Geometry check sheet. Reference: the model listing, model coordinates, mm. Coordinates: 2 decimals unless noted, no trailing zeros. Write each loop counter-clockwise with the first axis right and the second up, starting at its lowest first coordinate (ties: lowest second). Pieces come first, ordered by that corner, then holes. Notation, with made-up numbers: (33.5, -6.5) -> (53.5, -6.5) arc R23 cw to (53.5, 31.5) -> close; hole circle Ø11 at (87.25, -0.75). An arc over 180 degrees is marked (long way). One line per question, with ' | ' between items.
from build123d import *

# Parameters (mm, degrees)
KREISMUSTER1_COUNT = 15


with BuildPart() as part:
    # Skizze1 → Rotation1 (revolve)
    with BuildSketch(Plane.XY, mode=Mode.PRIVATE) as rotation1_sk:
        Polygon((16.14475863, 0), (16.14475863, 8.608081897), (23.261403386, 8.608081897), (28.845024076, 5.234644397), (28.845024076, 0), align=None)
    revolve(rotation1_sk.sketch.rotate(Axis((0, 0, 0), (0, 1, 0)), 90), axis=Axis((0, 0, 0), (0, 1, 0)))  # turned: the seam where the file's is

    # Skizze2 → Schnitt-Rotation1 (revolve, cut)
    with BuildSketch(Plane.XY):
        Polygon((18.433980943, 12.441833146), (35.219041201, 3.611138793), (33.767638602, 0.852365915), (16.982578344, 9.683060267), align=None)
    schnitt_rotation1 = revolve(axis=Axis((14.262929412, 14.636241782, 0), (0.884995308, -0.465599941, 0)), mode=Mode.SUBTRACT)

    # Kreismuster1: Schnitt-Rotation1 ×15 about axis
    kreismuster1_axis = Axis((0, 0, 0), (0, -1, 0))
    for i in range(1, KREISMUSTER1_COUNT):
        add(schnitt_rotation1.rotate(kreismuster1_axis, i * 360 / KREISMUSTER1_COUNT), mode=Mode.SUBTRACT)


solid = part.part
1. Material ranges on line 1 (Z direction, x = 7.5, y = 5.5); line 2 (X direction, y = 6.75, z = 0); line 3 (X direction, y = 2.25, z = -11), recorded low to high. Write a range as from..to.
Worked answers:
line 1: -23.8..-14.3, 14.3..23.8 | line 2: -26.34..-16.14, 16.14..22.56 | line 3: -26.67..-11.82, 11.82..26.67
2. Cross-section at A-A on z = 0. Record the boundary of the cut face in (x, y).
Worked answers:
outline: (-28.85, 0) -> (-16.14, 0) -> (-16.14, 8.61) -> (-23.26, 8.61) -> (-28.85, 5.23) -> close; (16.14, 0) -> (28.85, 0) -> (28.85, 3.44) -> (19.03, 8.61) -> (16.14, 8.61) -> close
3. Cross-section at B-B on y = 1. Record the boundary of the cut face in (x, z), and give its area (3 significant figures).
Worked answers:
outline: circle Ø57.69 at (0, 0); hole circle Ø32.29 at (0, 0) | area: 1,800 mm²
4. Mould release check, pull along Z, two halves, no side actions. Record for faces 1 (the face through (12, 0, -12)), 2 (the face through (25.53, 6.9, -5.38)), 3 (the face through (13.009, 6.898, 22.618)), 4 (the face through (-23.335, 6.062, -5.012)): released by +Z, released by -Z, zero draft, split by the parting line, or undercut.
Worked answers:
face 1: zero draft | face 2: released by -Z | face 3: released by +Z | face 4: undercut
